from build123d import *

# Parameters (mm, degrees)
SKETCH_W        = 47
SKETCH_H        = 50
SKETCH_R        = 10
SKETCH_R_2      = 1.5
PAD_DEPTH       = 2
SKETCH001_R     = 1.5
PAD001_DEPTH    = 2
SKETCH002_R     = 1.5
PAD002_DEPTH    = 8
SKETCH004_R     = 1.5
POCKET_DEPTH    = 8
PAD003_DEPTH    = 8
SKETCH005_R     = 1.5
POCKET001_DEPTH = 4
SKETCH006_R     = 1.5
SKETCH006_R_2   = 3.5
PAD004_DEPTH    = 2
SKETCH007_R     = 1.5
PAD005_DEPTH    = 8
SKETCH008_R     = 1.5
POCKET002_DEPTH = 8
PAD006_DEPTH    = 8
SKETCH010_R     = 1.5
POCKET003_DEPTH = 4
FILLET_R        = 3


with BuildPart() as part:
    # Sketch → Pad (new body)
    with BuildSketch(Plane.XY):
        Rectangle(SKETCH_W, SKETCH_H)
        Circle(SKETCH_R, mode=Mode.SUBTRACT)
        with Locations((-20, -19)):
            Circle(SKETCH_R_2, mode=Mode.SUBTRACT)
        with Locations((20, -19)):
            Circle(SKETCH_R_2, mode=Mode.SUBTRACT)
        with Locations((-20, 19)):
            Circle(SKETCH_R_2, mode=Mode.SUBTRACT)
        with Locations((20, 19)):
            Circle(SKETCH_R_2, mode=Mode.SUBTRACT)
    extrude(amount=PAD_DEPTH)

    # Sketch001 (on Face2 of Pad) → Pad001 (join)
    with BuildSketch(Plane.YZ.offset(23.5)):
        with BuildLine():
            Line((-25, 2), (25, 2))
            Line((25, -8), (25, 2))
            Line((22.505468, -27.843823), (25, -8))
            ThreePointArc((1.953944, -32.406741), (13.581707, -36.214738), (22.505468, -27.843823))
            Line((-13, -12.372281), (1.953944, -32.406741))
            ThreePointArc((-18.5, -9.5), (-16.620185, -12.602418), (-13, -12.372281))
            Line((-18.5, -8), (-18.5, -9.5))
            ThreePointArc((-18.5, -8), (-20.847064, -4.279548), (-25, -2.829168))
            Line((-25, 2), (-25, -2.829168))
        make_face()
        with Locations((-15, -9.5)):
            Circle(SKETCH001_R, mode=Mode.SUBTRACT)
        with Locations((15.980762, -19.5)):
            Circle(SKETCH001_R, mode=Mode.SUBTRACT)
        with Locations((5.980762, -19.5)):
            Circle(SKETCH001_R, mode=Mode.SUBTRACT)
        with Locations((10.980762, -24.5)):
            Circle(SKETCH001_R, mode=Mode.SUBTRACT)
        with Locations((15.980762, -29.5)):
            Circle(SKETCH001_R, mode=Mode.SUBTRACT)
        with Locations((5.980762, -29.5)):
            Circle(SKETCH001_R, mode=Mode.SUBTRACT)
    extrude(amount=PAD001_DEPTH)

    # Sketch002 (on Face9 of Pad001) → Pad002 (join)
    with BuildSketch(Plane(origin=(23.5, 0, 0), x_dir=(0, -1, 0), z_dir=(-1, 0, 0))):
        with BuildLine():
            Line((18.5, -8), (18.5, -9.5))
            ThreePointArc((11.5, -9.5), (15, -13), (18.5, -9.5))
            Line((11.5, -9.5), (11.5, 0))
            Line((25, 0), (11.5, 0))
            Line((25, 0), (25, -2.829168))
            ThreePointArc((25, -2.829168), (20.847064, -4.279548), (18.5, -8))
        make_face()
        with Locations((15, -9.5)):
            Circle(SKETCH002_R, mode=Mode.SUBTRACT)
    extrude(amount=PAD002_DEPTH)

    # Sketch004 (on Face35 of Pad002) → Pocket (cut)
    with BuildSketch(Plane.XY):
        with Locations((20, -19)):
            Circle(SKETCH004_R)
    extrude(amount=-POCKET_DEPTH, mode=Mode.SUBTRACT)

    # Sketch003 (on Face9 of Pad002) → Pad003 (join)
    with BuildSketch(Plane(origin=(23.5, 0, 0), x_dir=(0, -1, 0), z_dir=(-1, 0, 0))):
        with BuildLine():
            Line((-25, 0), (-15.5, 0))
            Line((-15.5, 0), (-15.5, -2))
            ThreePointArc((-17.5, -4), (-16.085786, -3.414214), (-15.5, -2))
            Line((-17.5, -4), (-22.5, -4))
            ThreePointArc((-25, -1.5), (-24.267767, -3.267767), (-22.5, -4))
            Line((-25, 0), (-25, -1.5))
        make_face()
    extrude(amount=PAD003_DEPTH)

    # Sketch005 (on Face41 of Pad003) → Pocket001 (cut)
    with BuildSketch(Plane.XY):
        with Locations((20, 19)):
            Circle(SKETCH005_R)
    extrude(amount=-POCKET001_DEPTH, mode=Mode.SUBTRACT)

    # Sketch006 (on Face2 of Pocket001) → Pad004 (join)
    with BuildSketch(Plane(origin=(-23.5, 0, 0), x_dir=(0, -1, 0), z_dir=(-1, 0, 0))):
        with BuildLine():
            Line((25, 2), (-25, 2))
            Line((-25, 2), (-25, -8))
            Line((-25, -8), (-22.505468, -27.843823))
            ThreePointArc((-22.505468, -27.843823), (-13.581707, -36.214738), (-1.953944, -32.406741))
            Line((-1.953944, -32.406741), (13, -12.372281))
            ThreePointArc((13, -12.372281), (16.620185, -12.602418), (18.5, -9.5))
            Line((18.5, -9.5), (18.5, -8))
            ThreePointArc((25, -2.829168), (20.847064, -4.279548), (18.5, -8))
            Line((25, -2.829168), (25, 2))
        make_face()
        with Locations((15, -9.5)):
            Circle(SKETCH006_R, mode=Mode.SUBTRACT)
        with Locations((-10.980762, -24.5)):
            Circle(SKETCH006_R_2, mode=Mode.SUBTRACT)
    extrude(amount=PAD004_DEPTH)

    # Sketch007 (on Face9 of Pad004) → Pad005 (join)
    with BuildSketch(Plane.YZ.offset(-23.5)):
        with BuildLine():
            Line((-11.5, 0), (-25, 0))
            Line((-25, 0), (-25, -2.829168))
            ThreePointArc((-18.5, -8), (-20.847064, -4.279548), (-25, -2.829168))
            Line((-18.5, -8), (-18.5, -9.5))
            ThreePointArc((-18.5, -9.5), (-15, -13), (-11.5, -9.5))
            Line((-11.5, 0), (-11.5, -9.5))
        make_face()
        with Locations((-15, -9.5)):
            Circle(SKETCH007_R, mode=Mode.SUBTRACT)
    extrude(amount=PAD005_DEPTH)

    # Sketch008 (on Face62 of Pad005) → Pocket002 (cut)
    with BuildSketch(Plane.XY):
        with Locations((-20, -19)):
            Circle(SKETCH008_R)
    extrude(amount=-POCKET002_DEPTH, mode=Mode.SUBTRACT)

    # Sketch009 (on Face9 of Pocket002) → Pad006 (join)
    with BuildSketch(Plane.YZ.offset(-23.5)):
        with BuildLine():
            Line((25, 0), (15.5, 0))
            Line((15.5, 0), (15.5, -2))
            ThreePointArc((15.5, -2), (16.085786, -3.414214), (17.5, -4))
            Line((17.5, -4), (22.5, -4))
            ThreePointArc((22.5, -4), (24.267767, -3.267767), (25, -1.5))
            Line((25, -1.5), (25, 0))
        make_face()
    extrude(amount=PAD006_DEPTH)

    # Sketch010 (on Face67 of Pad006) → Pocket003 (cut)
    with BuildSketch(Plane.XY):
        with Locations((-20, 19)):
            Circle(SKETCH010_R)
    extrude(amount=-POCKET003_DEPTH, mode=Mode.SUBTRACT)

    # Fillet
    fillet_edges = [part.edges().sort_by_distance(p)[0] for p in [
        (-19.5, -25, -2.829168),
        (-24.5, -25, -2.829168),
        (19.5, -25, -2.829168),
        (24.5, -25, -2.829168),
    ]]
    fillet(fillet_edges, radius=FILLET_R)


solid = part.part
Can you work these out from the model? Positions are in its coordinate system, mm. A direction names the side the tool comes from. Round coordinates to 2 decimals unless told otherwise and drop trailing zeros. Loops run counter-clockwise (first coordinate to the right, second up) from the corner with the lowest first, then second, coordinate; pieces in that order, holes last. Notation, with made-up numbers: (85, 68) - (115, 68) arc R26 ccw to (115, 88) - close; hole circle Ø4 at (2.5, 23). An arc over 180 degrees is marked (long way). Write item = value, one per line. Start each with the question number.
(1) If we section it at B-B (z = -19.5): Please give me the cut outline in (x, y).
(2) If we section it at D-D (y = 6): Please give me the cut outline in (x, z).
(3) For P1, Ø3.5, axis at x = -20, y = -19, coming from the -Z side; P2, Ø4, axis at x = -17.5, z = -6.5, coming from the +Y side; P3, Ø5, axis at x = 20, y = -19, coming from the +Z side; P4, Ø2.5, axis at y = 5.98, z = -19.5, coming from the +X side, each with a flat end and sliding along its axis, tell me the tip position at first contact or that it passes through.
(4) For faces 1 (the face through (20, 21, -4)), 2 (the face through (-20, 15.5, -1)), 3 (the face through (24.486, 14.875, -18.486)), 4 (the face through (-24.49, 7.64, -23.45)), which set-ups out of +Z, -Z, +X, -X, +Y, -Y let a thin tool reach every point of the face, with its end or its side?
(5) If we mould it in two halves opening along Y, with no side actions, what happens to faces 5 (the face through (20, -11.5, -5)), 6 (the face through (0, -11, 2)), 7 (the face through (-19.556, 24.248, -3.287))? For each: released by +Y, released by -Y, zero draft, split by the parting line, or undercut.
(6) If we section it at C-C (x = 0): Please give me the cut outline in (y, z), and give its area (3 significant figures).
(7) If I drill on probe 1 along X at (y, z) = (19, -1); probe 2 along X at (y, z) = (15, -4.5); probe 3 along Y at (x, z) = (0, 1.6), over which ranges is the centre line in solid material (lowest first)? Write a range as [from, to].
(8) If we section it at A-A (x = 17.5): Please give me the cut outline in (y, z), and give its area (3 significant figures).
Ans:
q1.outline = (-25.5, -7.68) - (-23.5, -7.68) - (-23.5, 23.55) - (-25.5, 23.55) - close; (23.5, -7.68) - (25.5, -7.68) - (25.5, 4.48) - (23.5, 4.48) - close; (23.5, 7.48) - (25.5, 7.48) - (25.5, 14.48) - (23.5, 14.48) - close; (23.5, 17.48) - (25.5, 17.48) - (25.5, 23.55) - (23.5, 23.55) - close
q2.outline = (-25.5, -35.42) - (-23.5, -35.42) - (-23.5, 0) - (-8, 0) - (-8, 2) - (-25.5, 2) - close; (8, 0) - (23.5, 0) - (23.5, -18) - (25.5, -18) - (25.5, 2) - (8, 2) - close; (23.5, -35.42) - (25.5, -35.42) - (25.5, -31) - (23.5, -31) - close; (23.5, -28) - (25.5, -28) - (25.5, -21) - (23.5, -21) - close
q3.P1 = -12.18
q3.P2 = -11.5
q3.P3 = 2
q3.P4 = -23.5
q4.face_1 = -Z, +Y
q4.face_2 = -Z
q4.face_3 = +X
q4.face_4 = -X
q5.face_5 = undercut
q5.face_6 = zero draft
q5.face_7 = released by +Y
q6.outline = (-25, 0) - (-10, 0) - (-10, 2) - (-25, 2) - close; (10, 0) - (25, 0) - (25, 2) - (10, 2) - close
q6.area = 60.0 mm²
q7.probe_1 = [-25.5, -21.5], [-18.5, -15.5], [15.5, 18.5], [21.5, 25.5]
q7.probe_2 = [-25.5, -23.5], [23.5, 25.5]
q7.probe_3 = [-25, -10], [10, 25]
q8.outline = (-25, -0.31) arc R3 ccw to (-22.93, -3.16) arc R6.67 cw to (-18.5, -8) - (-18.5, -9.5) arc R3.5 ccw to (-11.5, -9.5) - (-11.5, 0) - (15.5, 0) - (15.5, -2) arc R2 ccw to (17.5, -4) - (22.5, -4) arc R2.5 ccw to (25, -1.5) - (25, 2) - (-25, 2) - close; hole circle Ø3 at (-15, -9.5)
q8.area = 240 mm²
